The listing builds one solid part. Answer for the finished solid, in the listing's coordinates (mm). A direction names the side the tool comes from. Give positions to 0.01 mm unless a question says otherwise; leave off trailing zeros. Write each loop counter-clockwise with the first axis right and the second up, starting at its lowest first coordinate (ties: lowest second). Pieces come first, ordered by that corner, then holes. Notation, with made-up numbers: (13.25, -28) -> (18.25, -28) arc R9 ccw to (18.25, -23) -> close; hole circle Ø10 at (78.25, -7). An arc over 180 degrees is marked (long way). One line per question, with ' | ' between items.
from build123d import *


with BuildPart() as part:
    # Balayage1: sweep along a path in Esquisse1
    with BuildLine(Plane.XY) as balayage1_path:
        Line((0, 0), (0, 300))
        Line((0, 300), (600, 300))
        Line((600, 300), (600, 0))
    # Esquisse2 → Balayage1 (sweep)
    with BuildSketch(Plane(origin=(0, 0, 0), x_dir=(1, 0, 0), z_dir=(0, 1, 0))):
        with BuildLine():
            Line((-12, -15), (12, -15))
            ThreePointArc((12, -15), (14.121320344, -14.121320344), (15, -12))
            Line((15, -12), (15, 12))
            ThreePointArc((15, 12), (14.121320344, 14.121320344), (12, 15))
            Line((12, 15), (-12, 15))
            ThreePointArc((-12, 15), (-14.121320344, 14.121320344), (-15, 12))
            Line((-15, 12), (-15, -12))
            ThreePointArc((-15, -12), (-14.121320344, -14.121320344), (-12, -15))
        make_face()
        with BuildLine():
            Line((-10, -13), (10, -13))
            ThreePointArc((10, -13), (12.121320344, -12.121320344), (13, -10))
            Line((13, -10), (13, 10))
            ThreePointArc((13, 10), (12.121320344, 12.121320344), (10, 13))
            Line((10, 13), (-10, 13))
            ThreePointArc((-10, 13), (-12.121320344, 12.121320344), (-13, 10))
            Line((-13, 10), (-13, -10))
            ThreePointArc((-13, -10), (-12.121320344, -12.121320344), (-10, -13))
        make_face(mode=Mode.SUBTRACT)
    sweep(path=balayage1_path.line, transition=Transition.RIGHT)


solid = part.part
Item 1: Find section B-B (z = 2.5). Write down the section's boundary in (x, y), then the cut area to 3 significant figures.
Answers below:
outline: (-15, 0) -> (-13, 0) -> (-13, 313) -> (613, 313) -> (613, 0) -> (615, 0) -> (615, 315) -> (-15, 315) -> close; (13, 0) -> (15, 0) -> (15, 285) -> (585, 285) -> (585, 0) -> (587, 0) -> (587, 287) -> (13, 287) -> close | area: 4,800 mm²
Item 2: Find section C-C (x = 208). Write down the section's boundary in (y, z), then the cut area to 3 significant figures.
Answers below:
outline: (285, -12) arc R3 ccw to (288, -15) -> (312, -15) arc R3 ccw to (315, -12) -> (315, 12) arc R3 ccw to (312, 15) -> (288, 15) arc R3 ccw to (285, 12) -> close; hole (287, -10) arc R3 ccw to (290, -13) -> (310, -13) arc R3 ccw to (313, -10) -> (313, 10) arc R3 ccw to (310, 13) -> (290, 13) arc R3 ccw to (287, 10) -> close | area: 224 mm²
Item 3: A flat-ended cylindrical pin translates along its axis: pin 1 (6 mm diameter, centred on x = 178, z = -1.5, fed in from -Y). Find the tip coordinate at first contact, or state that the pin passes through.
Answers below:
pin 1: y = 285
Item 4: Consider line 1 (X direction, y = 22.5, z = 3); line 2 (Y direction, x = 79.5, z = -3.5); line 3 (X direction, y = 250, z = 12). Determine where each line is inside the solid, lowest interval first. Write a range as [from, to].
Answers below:
line 1: [-15, -13], [13, 15], [585, 587], [613, 615] | line 2: [285, 287], [313, 315] | line 3: [-15, -12.24], [12.24, 15], [585, 587.76], [612.24, 615]
Item 5: Find section A-A (y = 159). Count the separate pieces of the cut face and the enclosed holes in it, then the cut area to 3 significant figures.
Answers below:
separate pieces: 2 | enclosed holes: 2 | area: 448 mm²
Item 6: Determine the mould class of faces 1 (the face through (276, 294, -13)), 2 (the face through (275, 295, 15)), 3 (the face through (324, 294, 13)), 4 (the face through (-15, 160, 0)) for opening direction X: pulls with the +X half, pulls with the -X half, needs draft (parallel to the pull), parting line crosses it, or undercut.
Answers below:
face 1: undercut | face 2: needs draft | face 3: undercut | face 4: pulls with the -X half
Item 7: A tool of negligible diameter and unlimited length cuts with its end or side. For faces 5 (the face through (614, 0, 0)), 6 (the face through (-13, 159, 0)), 7 (the face through (585, 141, 0)), 8 (the face through (615, 155, 0)), 9 (the face through (304, 287, 0)), from which of +Z, -Z, +X, -X, +Y, -Y can it reach the whole face along a straight path? Write none if from no direction.
Answers below:
face 5: +Z, -Z, +X, -X, -Y | face 6: -Y | face 7: +Z, -Z, -Y | face 8: +Z, -Z, +X, +Y, -Y | face 9: none
